The listing builds one solid part. Answer for the finished solid, in the listing's coordinates (mm). Coordinates: 2 decimals unless noted, no trailing zeros. Order: outer loops, then holes, each group sorted by start corner. A loop starts at its lowest first (then second) coordinate and runs counter-clockwise, first axis right, second up. Notation, with made-up numbers: (77.25, 13.25) -> (131.25, 13.25) arc R15 ccw to (131.25, 22.25) -> close; hole circle Ø6 at (53.5, 42.25). An arc over 180 degrees is marked (long way). Return JSON: item names as keys, results as strings.
from build123d import *

# Parameters (mm, degrees)
SALIENTE_EXTRUIR1_DEPTH = 1.4


with BuildPart() as part:
    # Croquis1 → Saliente-Extruir1 (new body)
    with BuildSketch(Plane.XY):
        with BuildLine():
            Line((2.8, 4), (-1, 4))
            ThreePointArc((-1, 4), (-3.121320344, 3.121320344), (-4, 1))
            Line((-4, 1), (-4, -2.8))
            Line((-4, -2.8), (-2.628688939, -2.8))
            ThreePointArc((-2.628688939, -2.8), (-2.110290924, -2.468813544), (-2.192918912, -1.859228778))
            ThreePointArc((-2.192918912, -1.859228778), (-2.032931996, 2.032931996), (1.859228778, 2.192918912))
            ThreePointArc((1.859228778, 2.192918912), (2.468813544, 2.110290924), (2.8, 2.628688939))
            Line((2.8, 2.628688939), (2.8, 4))
        make_face()
    extrude(amount=SALIENTE_EXTRUIR1_DEPTH)


solid = part.part
1. The part is cut by section D-D on x = -3.25. Give the vertices of the cut face in (y, z), and give its area (3 significant figures).
Answer block:
{"outline": "(-2.8, 0) -> (2.98, 0) -> (2.98, 1.4) -> (-2.8, 1.4) -> close", "area": "8.10 mm2"}
2. The part is cut by section C-C on z = 0.8. Give the vertices of the cut face in (x, y) (3 decimals).
Answer block:
{"outline": "(-4, -2.8) -> (-2.629, -2.8) arc R0.571 ccw to (-2.193, -1.859) arc R2.875 cw to (1.859, 2.193) arc R0.571 ccw to (2.8, 2.629) -> (2.8, 4) -> (-1, 4) arc R3 ccw to (-4, 1) -> close"}
3. The part is cut by section A-A on y = 2.75. Give the vertices of the cut face in (x, z), and give its area (3 significant figures).
Answer block:
{"outline": "(-3.44, 0) -> (-0.84, 0) -> (-0.84, 1.4) -> (-3.44, 1.4) -> close; (0.84, 0) -> (2.8, 0) -> (2.8, 1.4) -> (0.84, 1.4) -> close", "area": "6.38 mm2"}
4. Determine the mould class of faces 1 (the face through (-2.2, 2.2, 0)), 2 (the face through (-2.114, -2.477, 0.69)), 3 (the face through (1, 4, 1)) for opening direction Y: pulls with the +Y half, pulls with the -Y half, needs draft (parallel to the pull), parting line crosses it, or undercut.
Answer block:
{"face 1": "needs draft", "face 2": "undercut", "face 3": "pulls with the +Y half"}
5. Consider line 1 (X direction, y = 0, z = 0.4) (3 decimals); line 2 (X direction, y = 2.5, z = 1.2); line 3 (Y direction, x = 0, z = 0.3) (3 decimals). Determine where each line is inside the solid, lowest interval first. Write a range as from..to.
Answer block:
{"line 1": "x = -4..-2.875", "line 2": "x = -3.6..-1.42, 1.42..2.79", "line 3": "y = 2.875..4"}
6. The part is cut by section B-B on y = 0. Give the vertices of the cut face in (x, z) (3 decimals).
Answer block:
{"outline": "(-4, 0) -> (-2.875, 0) -> (-2.875, 1.4) -> (-4, 1.4) -> close"}
